Source: CAD feature listing. Evaluate the final solid. Frame: model axes, mm. A direction names the side the tool comes from. Give positions to 0.01 mm unless a question says otherwise; leave off trailing zeros. Loops run counter-clockwise (first coordinate to the right, second up) from the corner with the lowest first, then second, coordinate; pieces in that order, holes last.
from build123d import *

# Parameters (mm, degrees)
SKETCH1_W           = 144.7
SKETCH1_H           = 8
BOSS_EXTRUDE1_DEPTH = 115
SKETCH3_W           = 10
SKETCH3_H           = 18
BOSS_EXTRUDE2_DEPTH = 14
SKETCH4_W           = 18
SKETCH4_H           = 7
BOSS_EXTRUDE6_DEPTH = 65
BOSS_EXTRUDE7_DEPTH = 10
BOSS_EXTRUDE8_DEPTH = 10


with BuildPart() as part:
    # Sketch1 → Boss-Extrude1 (new body)
    with BuildSketch(Plane.XY):
        with Locations((34.899775573, 7.072761635)):
            Rectangle(SKETCH1_W, SKETCH1_H)
    extrude(amount=BOSS_EXTRUDE1_DEPTH)

    # Sketch3 → Boss-Extrude2 (add)
    with BuildSketch(Plane.XZ.offset(-3.072761635)):
        with Locations((-32.450224427, 77.5)):
            Rectangle(SKETCH3_W, SKETCH3_H)
    extrude(amount=BOSS_EXTRUDE2_DEPTH)

    # Sketch4 → Boss-Extrude6 (add)
    with BuildSketch(Plane.ZY.offset(37.450224427)):
        with Locations((77.5, -7.427238365)):
            Rectangle(SKETCH4_W, SKETCH4_H)
    extrude(amount=BOSS_EXTRUDE6_DEPTH)

    # Sketch5 → Boss-Extrude7 (add)
    with BuildSketch(Plane.XY.offset(86.5)):
        Polygon((-37.450224427, 3.072761635), (-27.450224427, 3.072761635), (-27.450224427, -3.927238365), (-27.450224427, -10.927238365), (-37.450224427, -10.927238365), (-37.450224427, -3.927238365), align=None)
    extrude(amount=BOSS_EXTRUDE7_DEPTH)

    # Sketch6 → Boss-Extrude8 (add)
    with BuildSketch(Plane(origin=(0, 0, 68.5), x_dir=(-1, 0, 0), z_dir=(0, 0, -1))):
        Polygon((37.450224427, 3.072761635), (27.450224427, 3.072761635), (27.450224427, -3.927238365), (27.450224427, -10.927238365), (37.450224427, -10.927238365), (37.450224427, -3.927238365), align=None)
    extrude(amount=BOSS_EXTRUDE8_DEPTH)


solid = part.part
1) Reachability of faces 1 (the flat face through (-32, -4, 58.5)), 2 (the flat face through (-32, -4, 96.5)), 3 (the flat face through (-69, -7, 68.5)), 4 (the flat face through (-69, -7, 86.5)) from +Z, -Z, +X, -X, +Y, -Y: full face, straight path, thin tool, end or side. Return the list, or none.
Checks:
face 1: -Z, +X, -X, -Y
face 2: +Z, +X, -X, -Y
face 3: -Z, -X, +Y, -Y
face 4: +Z, -X, +Y, -Y
2) Cut plane D-D (z = 9). Return loops of the section in (x, y), and give its area (3 significant figures).
Checks:
outline: (-37.45, 3.07) - (107.25, 3.07) - (107.25, 11.07) - (-37.45, 11.07) - close
area: 1,160 mm2
3) Ray query, probe 1 along X at (y, z) = (7.75, 17); probe 2 along Z at (x, y) = (-27.5, 0.75); probe 3 along X at (y, z) = (-6.5, 67.5). Return the intervals inside material, ascending.
Checks:
probe 1: x = -37.45 to 107.25
probe 2: z = 58.5 to 96.5
probe 3: x = -37.45 to -27.45
4) Cut plane C-C (x = 2). Return loops of the section in (y, z), and give its area (3 significant figures).
Checks:
outline: (3.07, 0) - (11.07, 0) - (11.07, 115) - (3.07, 115) - close
area: 920 mm2
5) Contact query for flat-ended pins moving along their axis: P1, Ø12, axis at x = -62, y = 2, coming from the -Z side; P2, Ø3, axis at x = -66.5, z = 81, coming from the +Y side; P3, Ø1.5, axis at y = 1.5, z = 28.5, coming from the +X side (3 decimals); P4, Ø11, axis at y = 0, z = 55, coming from the -X side. Output: stop coordinate, or through.
Checks:
P1: stops at z = 68.5
P2: stops at y = -3.93
P3: passes through
P4: stops at x = -37.45
6) Cut plane A-A (z = 92.5). Return loops of the section in (x, y).
Checks:
outline: (-37.45, -10.93) - (-27.45, -10.93) - (-27.45, 3.07) - (107.25, 3.07) - (107.25, 11.07) - (-37.45, 11.07) - close
7) Cut plane B-B (y = -6.25). Return loops of the section in (x, z).
Checks:
outline: (-102.45, 68.5) - (-37.45, 68.5) - (-37.45, 58.5) - (-27.45, 58.5) - (-27.45, 96.5) - (-37.45, 96.5) - (-37.45, 86.5) - (-102.45, 86.5) - close
